```python
from build123d import *

# Parameters (mm, degrees)
CROQUIS1_W              = 35
CROQUIS1_H              = 35
CROQUIS1_R              = 2.25
SALIENTE_EXTRUIR1_DEPTH = 2
REDONDEO1_R             = 5
CROQUIS2_R              = 1.5
CORTAR_EXTRUIR1_DEPTH   = 25.829418036


with BuildPart() as part:
    # Croquis1 → Saliente-Extruir1 (new body)
    with BuildSketch(Plane.XY):
        Rectangle(CROQUIS1_W, CROQUIS1_H)
        Circle(CROQUIS1_R, mode=Mode.SUBTRACT)
    extrude(amount=SALIENTE_EXTRUIR1_DEPTH)

    # Redondeo1
    redondeo1_edges = [part.edges().sort_by_distance(p)[0] for p in [
        (17.5, -17.5, 1),
        (-17.5, -17.5, 1),
        (-17.5, 17.5, 1),
        (17.5, 17.5, 1),
    ]]
    fillet(redondeo1_edges, radius=REDONDEO1_R)

    # Croquis2 → Cortar-Extruir1 (cut, through all)
    with BuildSketch(Plane.XY.offset(2)):
        with Locations((-12.5, 12.5)):
            Circle(CROQUIS2_R)
        with Locations((12.5, 12.5)):
            Circle(CROQUIS2_R)
        with Locations((12.5, -12.5)):
            Circle(CROQUIS2_R)
        with Locations((-12.5, -12.5)):
            Circle(CROQUIS2_R)
    extrude(amount=-CORTAR_EXTRUIR1_DEPTH, mode=Mode.SUBTRACT)


solid = part.part
```
Here's how the part is built. I have some questions about the finished solid (model axes, mm). Give positions to 0.01 mm unless a question says otherwise; leave off trailing zeros. Loops run counter-clockwise (first coordinate to the right, second up) from the corner with the lowest first, then second, coordinate; pieces in that order, holes last. Notation, with made-up numbers: (85, 7) -> (136, 7) arc R22 cw to (136, 34) -> close; hole circle Ø5 at (25.25, 37). An arc over 180 degrees is marked (long way). Use one line per item in the form item = value. Start each with the question number.
1) Please list where these lines run through material, in increasing order: line 1 along Y through (x, z) = (12.5, 0.75); line 2 along Y through (x, z) = (11.5, 0.4); line 3 along X through (y, z) = (2, 1.55).
2) Imagine slicing it at B-B (z = 1.15). Please give me the cut outline in (x, y), then the cut area to 3 significant figures.
3) Imagine slicing it at A-A (x = 0). Please give me the cut outline in (y, z), then the cut area to 3 significant figures.
4) Imagine slicing it at D-D (x = 11.5). Please give me the cut outline in (y, z), then the cut area to 3 significant figures.
5) Thinking about a two-plate mould opening in Y: for faces 1 (the face through (17.5, 0, 1)), 2 (the face through (11, 12.57, 1.01)), 3 (the face through (-16.07, -16, 1.01)), 4 (the face through (0, 17.5, 1)), which applies, +Y half, -Y half, draft (parallel to the pull), parting line (faces both ways), or undercut?
6) Imagine slicing it at C-C (y = 1). Please give me the cut outline in (x, z), then the cut area to 3 significant figures.
7) For P1, Ø5, axis at x = -11, y = 2, coming from the -Z side, with a flat end and sliding along its axis, tell me the tip position at first contact or that it passes through.
Check values:
q1.line_1 = -17.5 to -14, -11 to 11, 14 to 17.5
q1.line_2 = -17.5 to -13.62, -11.38 to 11.38, 13.62 to 17.5
q1.line_3 = -17.5 to -1.03, 1.03 to 17.5
q2.outline = (-17.5, -12.5) arc R5 ccw to (-12.5, -17.5) -> (12.5, -17.5) arc R5 ccw to (17.5, -12.5) -> (17.5, 12.5) arc R5 ccw to (12.5, 17.5) -> (-12.5, 17.5) arc R5 ccw to (-17.5, 12.5) -> close; hole circle Ø3 at (-12.5, -12.5); hole circle Ø3 at (-12.5, 12.5); hole circle Ø4.5 at (0, 0); hole circle Ø3 at (12.5, -12.5); hole circle Ø3 at (12.5, 12.5)
q2.area = 1,160 mm^2
q3.outline = (-17.5, 0) -> (-2.25, 0) -> (-2.25, 2) -> (-17.5, 2) -> close; (2.25, 0) -> (17.5, 0) -> (17.5, 2) -> (2.25, 2) -> close
q3.area = 61.0 mm^2
q4.outline = (-17.5, 0) -> (-13.62, 0) -> (-13.62, 2) -> (-17.5, 2) -> close; (-11.38, 0) -> (11.38, 0) -> (11.38, 2) -> (-11.38, 2) -> close; (13.62, 0) -> (17.5, 0) -> (17.5, 2) -> (13.62, 2) -> close
q4.area = 61.1 mm^2
q5.face_1 = draft
q5.face_2 = undercut
q5.face_3 = -Y half
q5.face_4 = +Y half
q6.outline = (-17.5, 0) -> (-2.02, 0) -> (-2.02, 2) -> (-17.5, 2) -> close; (2.02, 0) -> (17.5, 0) -> (17.5, 2) -> (2.02, 2) -> close
q6.area = 61.9 mm^2
q7.P1 = 0
